The listing builds one solid part. Answer for the finished solid, in the listing's coordinates (mm). Coordinates: 2 decimals unless noted, no trailing zeros. Loops run counter-clockwise (first coordinate to the right, second up) from the corner with the lowest first, then second, coordinate; pieces in that order, holes last. Notation, with made-up numbers: M -34,-28 L -23,-28 A8 cw -23,-22 Z; hole C 50,-34.75 d9. An arc over 180 degrees is marked long. Answer as a JSON object with one key per item and string values. Group by question number.
1. A cutting plane is placed at B-B on y = -51. Give the vertices of the cut face in (x, z) (3 decimals).
2. A cutting plane is placed at A-A on x = 0. Give the vertices of the cut face in (y, z) (1 decimal), and give its area (3 significant figures).
3. A cutting plane is placed at C-C on z = -1. Give the vertices of the cut face in (x, y) (1 decimal), and give its area (3 significant figures).
4. Determine the mould class of faces 1 (the face through (-47.242, -25.868, 0.044)), 2 (the face through (-1, -63.5, 0)), 3 (the face through (-51.875, -3.287, -2.946)) for opening direction Y: released by +Y, released by -Y, zero draft, split by the parting line, or undercut.
5. Straight lines are drawn through the part: L1, parallel to Y at x = 44, z = -1.25; L2, parallel to Y at x = -46, z = -1.5; L3, parallel to Y at x = 0, z = -0.5. For each, find the intervals that lie inside material, in ascending order.
6. A cutting plane is placed at D-D on y = -35. Give the vertices of the cut face in (x, z) (3 decimals).
from build123d import *

# Parameters (mm, degrees)
SKETCH2_W                   = 110.49
SKETCH2_H                   = 6.35
BOSS_EXTRUDE1_DEPTH         = 63.5
SKETCH3_R                   = 14.437499981
CUT_EXTRUDE1_DEPTH          = 85.407242136
CHAMFER1_SIZE               = 6.35
TAP_DRILL_FOR_M7X1_0_TAP1_D = 6
FILLET2_R                   = 0.762


with BuildPart() as part:
    # Sketch2 → Boss-Extrude1 (new body)
    with BuildSketch(Plane(origin=(0, 0, 0), x_dir=(1, 0, 0), z_dir=(0, 1, 0))):
        Rectangle(SKETCH2_W, SKETCH2_H)
    extrude(amount=-BOSS_EXTRUDE1_DEPTH)

    # Sketch3 → Cut-Extrude1 (cut, through all)
    with BuildSketch(Plane.XY.offset(3.175)):
        with Locations((0, -28.8150046)):
            Circle(SKETCH3_R)
    extrude(amount=-CUT_EXTRUDE1_DEPTH, mode=Mode.SUBTRACT)

    # Chamfer1
    chamfer1_edges = [part.edges().sort_by_distance(p)[0] for p in [
        (55.245, 0, 0),
        (-55.245, 0, 0),
    ]]
    chamfer(chamfer1_edges, length=CHAMFER1_SIZE)

    # Tap Drill for M7x1.0 Tap1 (through all)
    with Locations(Plane(origin=(0, 0, -3.175), x_dir=(-1, 0, 0), z_dir=(0, 0, -1))):
        with Locations((44.245, -26), (44.245, -51), (-44.245, -51), (-44.245, -26)):
            Hole(TAP_DRILL_FOR_M7X1_0_TAP1_D / 2)

    # Fillet2
    fillet2_edges = [part.edges().sort_by_distance(p)[0] for p in [
        (55.245, -63.5, 0),
        (0, -63.5, -3.175),
        (0, 0, 3.175),
        (0, 0, -3.175),
        (48.895, 0, 0),
        (-48.895, 0, 0),
        (52.07, -3.175, 3.175),
        (-52.07, -3.175, 3.175),
        (-55.245, -6.35, 0),
        (52.07, -3.175, -3.175),
        (-52.07, -3.175, -3.175),
        (55.245, -6.35, 0),
        (-55.245, -63.5, 0),
        (-55.245, -34.925, -3.175),
        (55.245, -34.925, -3.175),
        (55.245, -34.925, 3.175),
        (-55.245, -34.925, 3.175),
        (0, -63.5, 3.175),
    ]]
    fillet(fillet2_edges, radius=FILLET2_R)


solid = part.part
From the geometry:
{
 "1": {"outline": "M -55.245,-2.413 A0.762 ccw -54.483,-3.175 L -47.245,-3.175 L -47.245,3.175 L -54.483,3.175 A0.762 ccw -55.245,2.413 Z; M -41.245,-3.175 L 41.245,-3.175 L 41.245,3.175 L -41.245,3.175 Z; M 47.245,-3.175 L 54.483,-3.175 A0.762 ccw 55.245,-2.413 L 55.245,2.413 A0.762 ccw 54.483,3.175 L 47.245,3.175 Z"},
 "2": {"outline": "M -63.5,-2.4 A0.8 ccw -62.7,-3.2 L -43.3,-3.2 L -43.3,3.2 L -62.7,3.2 A0.8 ccw -63.5,2.4 Z; M -14.4,-3.2 L -0.8,-3.2 A0.8 ccw 0,-2.4 L 0,2.4 A0.8 ccw -0.8,3.2 L -14.4,3.2 Z", "area": "219 mm²"},
 "3": {"outline": "M -55.2,-62.7 A0.8 ccw -54.5,-63.5 L 54.5,-63.5 A0.8 ccw 55.2,-62.7 L 55.2,-6.7 A0.8 ccw 55,-6.1 L 49.1,-0.2 A0.8 ccw 48.6,0 L -48.6,0 A0.8 ccw -49.1,-0.2 L -55,-6.1 A0.8 ccw -55.2,-6.7 Z; hole C -44.2,-51 d6; hole C -44.2,-26 d6; hole C 0,-28.8 d28.9; hole C 44.2,-51 d6; hole C 44.2,-26 d6", "area": "6,210 mm²"},
 "4": {"face 1": "undercut", "face 2": "released by -Y", "face 3": "released by +Y"},
 "5": {"L1": "y = -63.5 to -53.99, -48.01 to -28.99, -23.01 to 0", "L2": "y = -63.5 to -53.43, -48.57 to -28.43, -23.57 to 0", "L3": "y = -63.5 to -43.25, -14.38 to 0"},
 "6": {"outline": "M -55.245,-2.413 A0.762 ccw -54.483,-3.175 L -13.046,-3.175 L -13.046,3.175 L -54.483,3.175 A0.762 ccw -55.245,2.413 Z; M 13.046,-3.175 L 54.483,-3.175 A0.762 ccw 55.245,-2.413 L 55.245,2.413 A0.762 ccw 54.483,3.175 L 13.046,3.175 Z"}
}
